from build123d import *

# Parameters (mm, degrees)
EXTRUDE_1_DEPTH     = 323.85
SKETCH_2_R          = 7.112
CUT_EXTRUDE_1_DEPTH = 329.755380278


with BuildPart() as part:
    # 草图1 → 凸台-拉伸1 (new body)
    with BuildSketch(Plane.XY):
        with BuildLine():
            Line((0, 0), (35.98, 0))
            ThreePointArc((35.98, 0), (37.883814298, 0.788585702), (38.6724, 2.6924))
            Line((38.6724, 2.6924), (38.6724, 36.5252))
            ThreePointArc((38.6724, 36.5252), (33.8972, 41.3004), (29.122, 36.5252))
            ThreePointArc((29.122, 36.5252), (30.4682, 35.179), (31.8144, 36.5252))
            ThreePointArc((31.8144, 36.5252), (33.8972, 38.608), (35.98, 36.5252))
            Line((35.98, 36.5252), (35.98, 2.6924))
            Line((35.98, 2.6924), (0, 2.6924))
            Line((0, 2.6924), (0, 36.5252))
            ThreePointArc((0, 36.5252), (2.0828, 38.608), (4.1656, 36.5252))
            ThreePointArc((4.1656, 36.5252), (5.5118, 35.179), (6.858, 36.5252))
            ThreePointArc((6.858, 36.5252), (2.0828, 41.3004), (-2.6924, 36.5252))
            Line((-2.6924, 36.5252), (-2.6924, 2.6924))
            ThreePointArc((-2.6924, 2.6924), (-1.903814298, 0.788585702), (0, 0))
        make_face()
    extrude(amount=EXTRUDE_1_DEPTH)

    # 草图2 → 切除-拉伸1 (cut, through all)
    with BuildSketch(Plane(origin=(0, 0, 0), x_dir=(-1, 0, 0), z_dir=(0, -1, 0))):
        with Locations(Location((-17.99, -28.448, 0), (0, 0, 90))):
            Circle(SKETCH_2_R)
        with Locations(Location((-17.99, -76.2, 0), (0, 0, 90))):
            Circle(SKETCH_2_R)
        with Locations(Location((-17.99, -295.402, 0), (0, 0, 90))):
            Circle(SKETCH_2_R)
        with Locations(Location((-17.99, -247.65, 0), (0, 0, 90))):
            Circle(SKETCH_2_R)
    extrude(amount=-CUT_EXTRUDE_1_DEPTH, mode=Mode.SUBTRACT)


solid = part.part
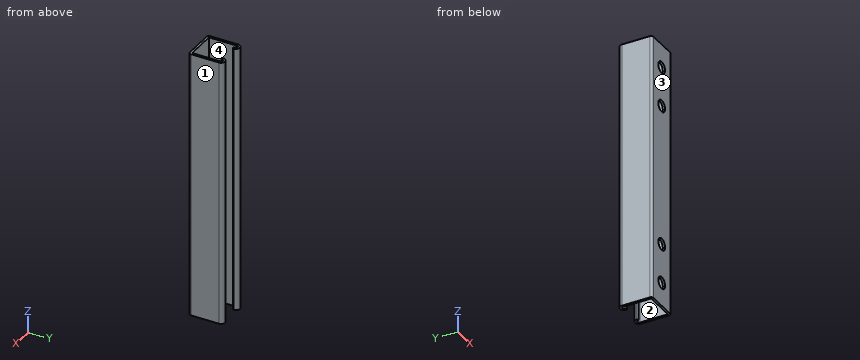
Design review of the part built by this model. Coordinates are the model's own, in mm. Face numbers are marked on the shaded views. Coordinates: 2 decimals unless noted, no trailing zeros. Loops run counter-clockwise (first coordinate to the right, second up) from the corner with the lowest first, then second, coordinate; pieces in that order, holes last. Notation, with made-up numbers: M 28.25,68 L 60.25,68 A34 ccw 60.25,105 Z; hole C 6,51 d11. An arc over 180 degrees is marked long. Use one line per item in the form item = value.
(1) Clearance check with a flat-ended pin moving along its axis: P1, Ø6, axis at x = 12.5, z = 39, coming from the +Y side. State where the tip first meets the part, or that it passes through.
Return value:
P1 = 2.69
(2) Draft analysis for pull direction Y (two halves, no side actions). For the marked faces 1, 2, 3 and 4, state which applies: pulls with the +Y half, pulls with the -Y half, needs draft (parallel to the pull), parting line crosses it, or undercut.
Return value:
face_1 = needs draft
face_2 = undercut
face_3 = pulls with the -Y half
face_4 = undercut
(3) Consider section C-C (y = 23.5). Write out the cut boundary in (x, z), and give its area (3 significant figures).
Return value:
outline = M -2.69,0 L 0,0 L 0,323.85 L -2.69,323.85 Z; M 35.98,0 L 38.67,0 L 38.67,323.85 L 35.98,323.85 Z
area = 1,740 mm2
(4) For line 1 along X through (y, z) = (11.5, 178); line 2 along X through (y, z) = (2.15, 76.2); line 3 along X through (y, z) = (38, 283), list the stretches that pass through material, from the lowest coordinate up. Write a range as from..to.
Return value:
line_1 = -2.69..0, 35.98..38.67
line_2 = -2.64..10.88, 25.1..38.62
line_3 = -2.46..0.61, 3.55..6.62, 29.36..32.43, 35.37..38.44
(5) Consider section B-B (x = 17.99). Write out the cut boundary in (y, z), and give its area (3 significant figures).
Return value:
outline = M 0,0 L 2.69,0 L 2.69,21.34 L 0,21.34 Z; M 0,35.56 L 2.69,35.56 L 2.69,69.09 L 0,69.09 Z; M 0,83.31 L 2.69,83.31 L 2.69,240.54 L 0,240.54 Z; M 0,254.76 L 2.69,254.76 L 2.69,288.29 L 0,288.29 Z; M 0,302.51 L 2.69,302.51 L 2.69,323.85 L 0,323.85 Z
area = 719 mm2
